Study the drawing (mm; zero at the part's minimum x, y, z) and answer. Give positions to 0.01 mm unless a question says otherwise; leave off trailing zeros. Loops run counter-clockwise (first coordinate to the right, second up) from the corner with the lowest first, then second, coordinate; pieces in that order, holes last. Notation, with made-up numbers: (85, -25) - (130, -25) arc R25 cw to (130, 14) - close; hole circle Ø10 at (51, 47.25). An arc over 180 degrees is marked (long way). One line per item, written item: value. Start each with the question number.
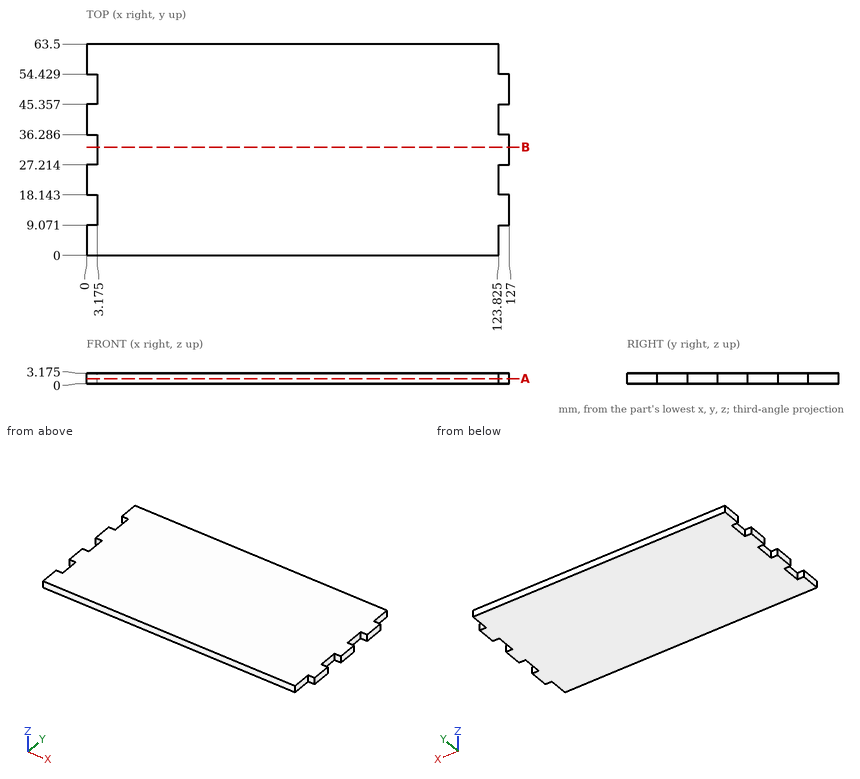
1. Find the intervals of material crossed by L1, parallel to X at y = 10.5, z = 0.6 (1 decimal); L2, parallel to X at y = 59, z = 1 (1 decimal), in increasing order. Write a range as [from, to].
2. Flat-ended cylindrical pins translate along their axes: pin 1 (1 mm diameter, centred on y = 61, z = 1.5, fed in from +X) (3 decimals); pin 2 (1.6 mm diameter, centred on x = 126, z = 1, fed in from +Y); pin 3 (1.6 mm diameter, centred on x = 126, z = 1, fed in from -Y). Find the tip coordinate at first contact, or state that the pin passes through.
3. A cutting plane is placed at A-A (z = 1.6). Determine the outline of the cut face in (x, y) (1 decimal), plus the area to 3 significant figures.
4. A cutting plane is placed at B-B (y = 32.5). Determine the outline of the cut face in (x, z) (1 decimal).
Results below:
1. L1: x = [3.2, 127]
1. L2: x = [0, 123.8]
2. pin 1: stops at x = 123.825
2. pin 2: stops at y = 54.43
2. pin 3: stops at y = 9.07
3. outline: (0, 0) - (123.8, 0) - (123.8, 9.1) - (127, 9.1) - (127, 18.1) - (123.8, 18.1) - (123.8, 27.2) - (127, 27.2) - (127, 36.3) - (123.8, 36.3) - (123.8, 45.4) - (127, 45.4) - (127, 54.4) - (123.8, 54.4) - (123.8, 63.5) - (0, 63.5) - (0, 54.4) - (3.2, 54.4) - (3.2, 45.4) - (0, 45.4) - (0, 36.3) - (3.2, 36.3) - (3.2, 27.2) - (0, 27.2) - (0, 18.1) - (3.2, 18.1) - (3.2, 9.1) - (0, 9.1) - close
3. area: 7,860 mm^2
4. outline: (3.2, 0) - (127, 0) - (127, 3.2) - (3.2, 3.2) - close
